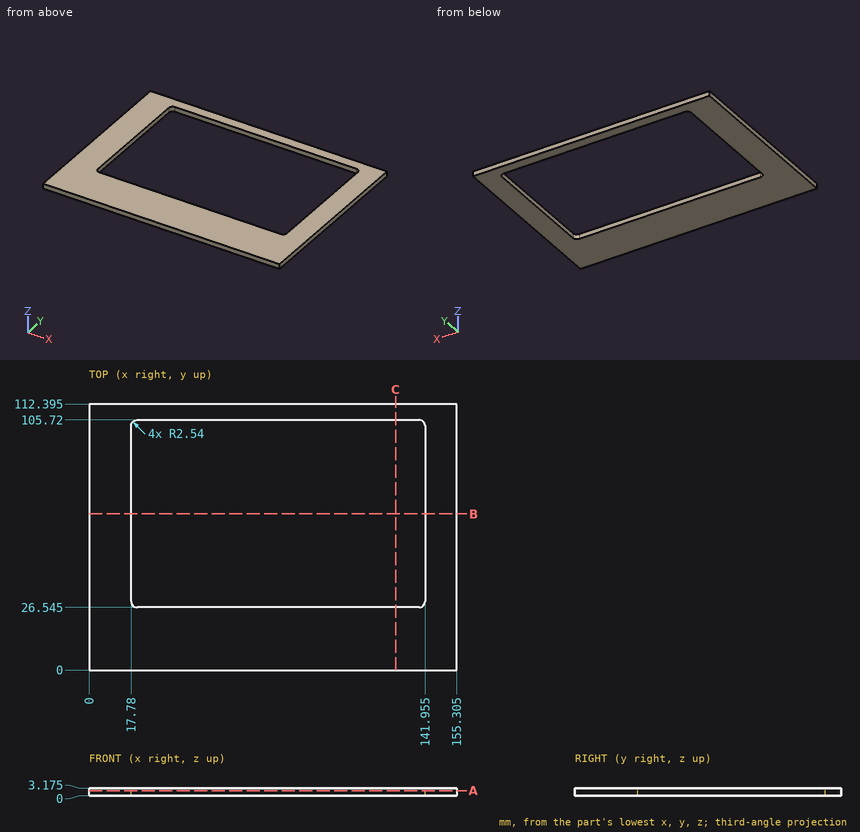
Study the drawing (mm; zero at the part's minimum x, y, z) and answer. Give positions to 0.01 mm unless a question says otherwise; leave off trailing zeros. Loops run counter-clockwise (first coordinate to the right, second up) from the corner with the lowest first, then second, coordinate; pieces in that order, holes last. Notation, with made-up numbers: (35, -35) - (51, -35) arc R26 ccw to (51, -3) - close; hole circle Ø3 at (-11, 45). An arc over 180 degrees is marked (long way). Answer as CSV lines item,"result". Start each with the question number.
1) Find section A-A (z = 2.1). Write down the section's boundary in (x, y) (3 decimals), then the cut area to 3 significant figures.
2) Find section B-B (y = 66). Write down the section's boundary in (x, z) (3 decimals), then the cut area to 3 significant figures.
3) Straight lines are drawn through the part: L1, parallel to Y at x = 38, z = 0.9 (3 decimals); L2, parallel to X at y = 89.5, z = 2.95 (3 decimals); L3, parallel to Y at x = 18.5, z = 2.65 (3 decimals). For each, find the intervals that lie inside material, in ascending order. Write a range as from..to.
4) Find section C-C (x = 129.5). Write down the section's boundary in (y, z) (3 decimals), then the cut area to 3 significant figures.
5) Each of these flat-tipped pins is pushed along its axis until it touches: pin 1 Ø8 at (x, y) = (34.5, 21.5) entering from -Z; pin 2 Ø8 at (x, y) = (68.5, 31.5) entering from +Z. Where does it stop, or does it pass through?
Findings below:
1,outline,"(0, 0) - (155.305, 0) - (155.305, 112.395) - (0, 112.395) - close; hole (17.78, 29.085) arc R2.54 ccw to (20.32, 26.545) - (139.415, 26.545) arc R2.54 ccw to (141.955, 29.085) - (141.955, 103.18) arc R2.54 ccw to (139.415, 105.72) - (20.32, 105.72) arc R2.54 ccw to (17.78, 103.18) - close"
1,area,"7,630 mm^2"
2,outline,"(0, 0) - (17.78, 0) - (17.78, 3.175) - (0, 3.175) - close; (141.955, 0) - (155.305, 0) - (155.305, 3.175) - (141.955, 3.175) - close"
2,area,"98.8 mm^2"
3,L1,"0..26.545, 105.72..112.395"
3,L2,"0..17.78, 141.955..155.305"
3,L3,"0..27.313, 104.952..112.395"
4,outline,"(0, 0) - (26.545, 0) - (26.545, 3.175) - (0, 3.175) - close; (105.72, 0) - (112.395, 0) - (112.395, 3.175) - (105.72, 3.175) - close"
4,area,"105 mm^2"
5,pin 1,"z = 0"
5,pin 2,"through"
